The listing builds one solid part. Answer for the finished solid, in the listing's coordinates (mm). Give positions to 0.01 mm unless a question says otherwise; leave off trailing zeros. Write each loop counter-clockwise with the first axis right and the second up, starting at its lowest first coordinate (ties: lowest second). Pieces come first, ordered by that corner, then holes. Notation, with made-up numbers: (16.5, 7.25) - (30.5, 7.25) arc R23 ccw to (30.5, 21.25) - close; hole circle Ø4 at (-27.5, -39.75). An arc over 180 degrees is marked (long way). Answer as CSV lines item,"result". Start each with the question number.
(1) For a pull along X with two mould halves and no side action, classify faces 1 (the face through (3.466, 3.955, 22.152)), 2 (the face through (0, 4, 67)), 3 (the face through (3.955, 4.501, 10.292)) as pulls with the +X half, pulls with the -X half, needs draft (parallel to the pull), parting line crosses it, or undercut.
(2) This flat-tipped pin is pushed along its axis until it touches: pin 1 Ø3.5 at (x, z) = (3.9, 20.2) entering from -Y. Where does it stop, or does it pass through?
(3) Find section B-B (y = 3.9). Write down the section's boundary in (x, z).
(4) Find section A-A (x = 3.9). Write down the section's boundary in (y, z).
(5) Find section C-C (z = 4.2). Write down the section's boundary in (x, y), then the cut area to 3 significant figures.
(6) Straight lines are drawn through the part: probe 1 along Z at (x, y) = (3.9, 1.75); probe 2 along Z at (x, y) = (3.9, 3.25); probe 3 along Z at (x, y) = (3.5, 5). For each, find the intervals that lie inside material, in ascending order.
Autodesk Inventor part; units mm, degrees
ref_plane "YZ Plane" through (0, 0, 0) normal (1, 0, 0) x (0, 1, 0)
ref_plane "XZ Plane" through (0, 0, 0) normal (0, 1, 0) x (-1, 0, 0)
ref_plane "XY Plane" through (0, 0, 0) normal (0, 0, 1) x (1, 0, 0)
sketch "Sketch1" plane through (0, 0, 0) normal (0, 0, 1) x (1, 0, 0)
  line L0 (0, 0) -> (7.8, 0)
  line L1 (7.8, 0) -> (7.8, 7.8)
  line L2 (7.8, 7.8) -> (0, 7.8)
  line L3 (0, 7.8) -> (0, 0)
  dimension "d0" = 7.8
  dimension "d1" = 7.8
extrude "Extrusion1" add sketch "Sketch1" along normal blind 136
sketch "Sketch2" plane through (0, 7.8, 0) normal (0, 1, 0) x (1, 0, 0)
  line L0 (0, 0) -> (3.9, 0)
  line L1 (7.8, 0) -> (0, 0)
  line L2 (3.9, 0) -> (3.9, -2.2)
  line L3 (3.9, -2.2) -> (3.9, -4.2)
  circle A0 centre (3.9, -4.2) radius 2
  dimension "d4" = 2.2
  dimension "d5" = 2
  dimension "d6" = 4
extrude "Extrusion2" cut sketch "Sketch2" against normal blind 136
sketch "Sketch3" plane through (7.8, 0, 0) normal (1, 0, 0) x (0, 0, -1)
  line L0 (0, 0) -> (0, 7.8)
  line L1 (0, 7.8) -> (0, 3.9)
  line L2 (0, 3.9) -> (-10.2, 3.9)
  line L3 (-10.2, 3.9) -> (-12.2, 3.9)
  circle A0 centre (-12.2, 3.9) radius 2
  dimension "d9" = 10.2
  dimension "d10" = 2
extrude "Extrusion3" cut sketch "Sketch3" against normal blind 136
sketch "Sketch4" plane through (0, 7.8, 0) normal (0, 1, 0) x (1, 0, 0)
  circle A0 centre (3.9, -4.2) radius 2
  line L0 (3.9, -6.2) -> (3.9, -8.4)
  line L1 (0, 0) -> (7.8, 0)
  line L2 (7.8, -10.2) -> (0, -10.2)
  line L3 (3.9, -8.4) -> (3.9, -10.4)
  line L4 (3.9, -6.2) -> (3.9, -18.2)
  line L5 (3.9, -18.2) -> (3.9, -20.2)
  circle A1 centre (3.9, -20.2) radius 2
  dimension "d13" = 2.2
  dimension "d15" = 2
  dimension "d16" = 12
  dimension "d17" = 2
extrude "Extrusion4" cut sketch "Sketch4" against normal blind 136 contours A1
ref_plane "Work Plane1" through (0, 0, 68) normal (0, 0, -1) x (-1, 0, 0)
ref_plane "Work Plane2" through (0, 3.9, 0) normal (0, 1, 0) x (1, 0, 0)
Result set:
1,face 1,"undercut"
1,face 2,"pulls with the -X half"
1,face 3,"needs draft"
2,pin 1,"through"
3,outline,"(0, 0) - (7.8, 0) - (7.8, 10.2) - (0, 10.2) - close; (0, 14.2) - (7.8, 14.2) - (7.8, 136) - (0, 136) - close; hole circle Ø4 at (3.9, 4.2); hole circle Ø4 at (3.9, 20.2)"
4,outline,"(0, 0) - (7.8, 0) - (7.8, 2.2) - (0, 2.2) - close; (0, 6.2) - (7.8, 6.2) - (7.8, 18.2) - (0, 18.2) - close; (0, 22.2) - (7.8, 22.2) - (7.8, 136) - (0, 136) - close; hole circle Ø4 at (3.9, 12.2)"
5,outline,"(0, 0) - (1.9, 0) - (1.9, 7.8) - (0, 7.8) - close; (5.9, 0) - (7.8, 0) - (7.8, 7.8) - (5.9, 7.8) - close"
5,area,"29.6 mm^2"
6,probe 1,"0 to 2.2, 6.2 to 18.2, 22.2 to 136"
6,probe 2,"0 to 2.2, 6.2 to 10.31, 14.09 to 18.2, 22.2 to 136"
6,probe 3,"0 to 2.24, 6.16 to 10.53, 13.87 to 18.24, 22.16 to 136"
